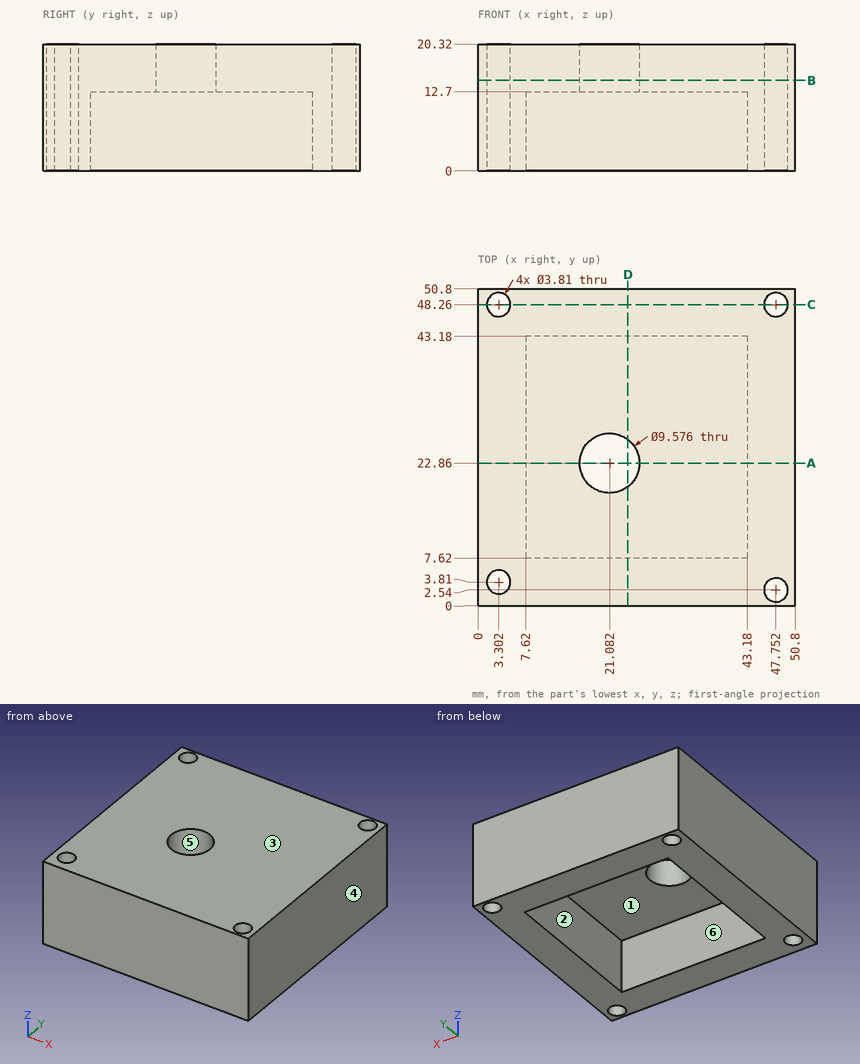
Could you check a few things on this drawing? It's one solid part, dimensions in mm from its lowest x, y, z. A direction names the side the tool comes from. Coordinates: 2 decimals unless noted, no trailing zeros. Write each loop counter-clockwise with the first axis right and the second up, starting at its lowest first coordinate (ties: lowest second). Pieces come first, ordered by that corner, then holes. Notation, with made-up numbers: (79, 13) - (88, 13) arc R17 cw to (88, 44) - close; hole circle Ø10 at (-27, 59). An arc over 180 degrees is marked (long way). Return JSON: item names as keys, results as strings. Group by question number.
Item 1: If we section it at B-B (z = 14.5): Write out the boundary of the cut face in (x, y) (1 decimal), then the cut area to 3 significant figures.
Item 2: We'd pull the mould along X, two halves only. Please class the marked faces 1, 2, 3 and 4: pulls with the +X half, pulls with the -X half, needs draft (parallel to the pull), parting line crosses it, or undercut.
Item 3: If we section it at A-A (y = 22.86): Write out the boundary of the cut face in (x, z).
Item 4: Which directions (+Z, -Z, +X, -X, +Y, -Y) give clear straight access to the entire face, cutting with the end or side of a thin tool? Please do the marked faces 5 and 6.
Item 5: If we section it at D-D (x = 24): Write out the boundary of the cut face in (y, z).
Item 6: If we section it at C-C (y = 48.26): Write out the boundary of the cut face in (x, z).
Item 7: I'm going to push a flat-ended pin straight in: pin 1 Ø10 at (x, y) = (21, 36) entering from -Z. Where does the tip first touch, or does it pass through?
Item 8: Please list where these lines run through material, in increasing order: probe 1 along X at (y, z) = (48.26, 16); probe 2 along X at (y, z) = (36, 10.75).
Return value:
{
 "1": {"outline": "(0, 0) - (50.8, 0) - (50.8, 50.8) - (0, 50.8) - close; hole circle Ø3.8 at (3.3, 3.8); hole circle Ø3.8 at (3.3, 48.3); hole circle Ø9.6 at (21.1, 22.9); hole circle Ø3.8 at (47.8, 2.5); hole circle Ø3.8 at (47.8, 48.3)", "area": "2,460 mm^2"},
 "2": {"face 1": "undercut", "face 2": "undercut", "face 3": "needs draft", "face 4": "pulls with the +X half"},
 "3": {"outline": "(0, 0) - (7.62, 0) - (7.62, 12.7) - (16.29, 12.7) - (16.29, 20.32) - (0, 20.32) - close; (25.87, 12.7) - (43.18, 12.7) - (43.18, 0) - (50.8, 0) - (50.8, 20.32) - (25.87, 20.32) - close"},
 "4": {"face 5": "+Z, -Z", "face 6": "-Z"},
 "5": {"outline": "(0, 0) - (7.62, 0) - (7.62, 12.7) - (19.06, 12.7) - (19.06, 20.32) - (0, 20.32) - close; (26.66, 12.7) - (43.18, 12.7) - (43.18, 0) - (50.8, 0) - (50.8, 20.32) - (26.66, 20.32) - close"},
 "6": {"outline": "(0, 0) - (1.4, 0) - (1.4, 20.32) - (0, 20.32) - close; (5.21, 0) - (45.85, 0) - (45.85, 20.32) - (5.21, 20.32) - close; (49.66, 0) - (50.8, 0) - (50.8, 20.32) - (49.66, 20.32) - close"},
 "7": {"pin 1": "stops at z = 12.7"},
 "8": {"probe 1": "x = 0 to 1.4, 5.21 to 45.85, 49.66 to 50.8", "probe 2": "x = 0 to 7.62, 43.18 to 50.8"}
}
